from build123d import *

# Parameters (mm, degrees)
SKETCH1_W           = 115
SKETCH1_H           = 69
BOSS_EXTRUDE1_DEPTH = 4
SKETCH2_R           = 2
CUT_EXTRUDE1_DEPTH  = 4
SKETCH3_W           = 90
SKETCH3_H           = 35
CUT_EXTRUDE2_DEPTH  = 4
CHAMFER1_SIZE       = 0.5
FILLET1_R           = 1.5


with BuildPart() as part:
    # Sketch1 → Boss-Extrude1 (new body)
    with BuildSketch(Plane.XY):
        Rectangle(SKETCH1_W, SKETCH1_H)
    extrude(amount=BOSS_EXTRUDE1_DEPTH)

    # Sketch2 → Cut-Extrude1 (cut)
    with BuildSketch(Plane.XY.offset(4)):
        with Locations((-35.5, 24.5)):
            Circle(SKETCH2_R)
        with Locations((39.5, 24.5)):
            Circle(SKETCH2_R)
        with Locations((46.979, -24.5)):
            Circle(SKETCH2_R)
        with Locations((-35.5, -24.5)):
            Circle(SKETCH2_R)
    extrude(amount=-CUT_EXTRUDE1_DEPTH, mode=Mode.SUBTRACT)

    # Sketch3 → Cut-Extrude2 (cut)
    with BuildSketch(Plane.XY.offset(4)):
        Rectangle(SKETCH3_W, SKETCH3_H)
    extrude(amount=-CUT_EXTRUDE2_DEPTH, mode=Mode.SUBTRACT)

    # Chamfer1
    chamfer1_edges = [part.edges().sort_by_distance(p)[0] for p in [
        (44.979, -24.5, 4),
        (-37.5, 24.5, 4),
        (-37.5, -24.5, 4),
        (37.5, 24.5, 4),
    ]]
    chamfer(chamfer1_edges, length=CHAMFER1_SIZE)

    # Fillet1
    fillet1_edges = [part.edges().sort_by_distance(p)[0] for p in [
        (-57.5, 0, 4),
        (0, -34.5, 4),
        (45, 0, 0),
        (45, 17.5, 2),
        (0, -17.5, 0),
        (-45, 0, 0),
        (-45, -17.5, 2),
        (0, 17.5, 0),
        (-45, 17.5, 2),
        (45, 0, 4),
        (0, 17.5, 4),
        (-45, 0, 4),
        (0, -17.5, 4),
        (57.5, 0, 4),
        (0, -34.5, 0),
        (-57.5, 0, 0),
        (0, 34.5, 0),
        (57.5, 0, 0),
        (57.5, -34.5, 2),
        (-57.5, -34.5, 2),
        (-57.5, 34.5, 2),
        (57.5, 34.5, 2),
        (0, 34.5, 4),
    ]]
    fillet(fillet1_edges, radius=FILLET1_R)


solid = part.part
Model file for the job. Use its own axes, mm. Give positions to 0.01 mm unless a question says otherwise; leave off trailing zeros. Loops run counter-clockwise (first coordinate to the right, second up) from the corner with the lowest first, then second, coordinate; pieces in that order, holes last.
Item 1: Drop flat-ended pins along their axis: P1, Ø2, axis at x = 12.5, y = 17, coming from the +Z side; P2, Ø1.5, axis at x = 15, z = 3.5, coming from the +Y side. Give the stop position or say it passes through.
Check values:
P1: stops at z = 3.62
P2: stops at y = 34.48
Item 2: Drill centre lines: line 1 along Y through (x, z) = (39.5, 1.6); line 2 along Y through (x, z) = (-35.5, 2.2); line 3 along X through (y, z) = (11.5, 2.25). Where is each one in solid material? Low to high.
Check values:
line 1: y = -34.5 to -17.5, 17.5 to 22.5, 26.5 to 34.5
line 2: y = -34.5 to -26.5, -22.5 to -17.5, 17.5 to 22.5, 26.5 to 34.5
line 3: x = -57.5 to -45, 45 to 57.5
Item 3: Mould opens along Y. For faces 1 (the face through (-1, 22, 0)), 2 (the face through (-33.653, 23.734, 1.774)) say: +Y half, -Y half, draft (parallel to the pull), parting line (faces both ways), or undercut.
Check values:
face 1: draft
face 2: undercut
Item 4: Slice it at B-B (x = 39.5). Write the cut outline in (y, z), plus the area to 3 significant figures.
Check values:
outline: (-34.5, 1.5) arc R1.5 ccw to (-33, 0) - (-19, 0) arc R1.5 ccw to (-17.5, 1.5) - (-17.5, 2.5) arc R1.5 ccw to (-19, 4) - (-33, 4) arc R1.5 ccw to (-34.5, 2.5) - close; (17.5, 1.5) arc R1.5 ccw to (19, 0) - (22.5, 0) - (22.5, 3.5) - (22, 4) - (19, 4) arc R1.5 ccw to (17.5, 2.5) - close; (26.5, 0) - (33, 0) arc R1.5 ccw to (34.5, 1.5) - (34.5, 2.5) arc R1.5 ccw to (33, 4) - (27, 4) - (26.5, 3.5) - close
area: 116 mm2
Item 5: Slice it at C-C (x = 18). Write the cut outline in (y, z), plus the area to 3 significant figures.
Check values:
outline: (-34.5, 1.5) arc R1.5 ccw to (-33, 0) - (-19, 0) arc R1.5 ccw to (-17.5, 1.5) - (-17.5, 2.5) arc R1.5 ccw to (-19, 4) - (-33, 4) arc R1.5 ccw to (-34.5, 2.5) - close; (17.5, 1.5) arc R1.5 ccw to (19, 0) - (33, 0) arc R1.5 ccw to (34.5, 1.5) - (34.5, 2.5) arc R1.5 ccw to (33, 4) - (19, 4) arc R1.5 ccw to (17.5, 2.5) - close
area: 132 mm2
Item 6: Slice it at D-D (y = 24.5). Write the cut outline in (x, z), plus the area to 3 significant figures.
Check values:
outline: (-57.5, 1.5) arc R1.5 ccw to (-56, 0) - (-37.5, 0) - (-37.5, 3.5) - (-38, 4) - (-56, 4) arc R1.5 ccw to (-57.5, 2.5) - close; (-33.5, 0) - (37.5, 0) - (37.5, 3.5) - (37, 4) - (-33, 4) - (-33.5, 3.5) - close; (41.5, 0) - (56, 0) arc R1.5 ccw to (57.5, 1.5) - (57.5, 2.5) arc R1.5 ccw to (56, 4) - (42, 4) - (41.5, 3.5) - close
area: 426 mm2
Item 7: Slice it at A-A (y = -5). Write the cut outline in (x, z).
Check values:
outline: (-57.5, 1.5) arc R1.5 ccw to (-56, 0) - (-46.5, 0) arc R1.5 ccw to (-45, 1.5) - (-45, 2.5) arc R1.5 ccw to (-46.5, 4) - (-56, 4) arc R1.5 ccw to (-57.5, 2.5) - close; (45, 1.5) arc R1.5 ccw to (46.5, 0) - (56, 0) arc R1.5 ccw to (57.5, 1.5) - (57.5, 2.5) arc R1.5 ccw to (56, 4) - (46.5, 4) arc R1.5 ccw to (45, 2.5) - close
